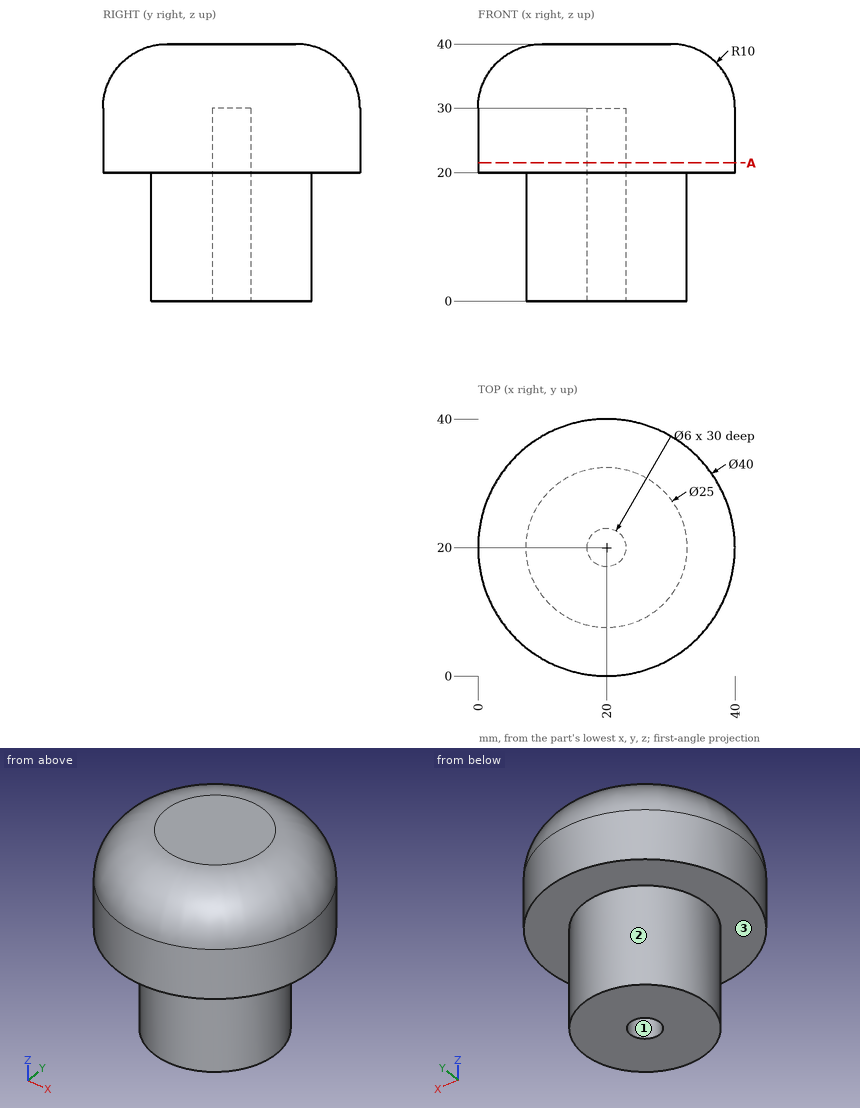
Answer from the drawing. Dimensions are ordinates in mm from the lowest x, y and z of the part. Give positions to 0.01 mm unless a question says otherwise; leave off trailing zeros. Order: outer loops, then holes, each group sorted by start corner. A loop starts at its lowest first (then second) coordinate and runs counter-clockwise, first axis right, second up. Notation, with made-up numbers: (80, 28.25) - (102, 28.25) arc R21 ccw to (102, 39.25) - close; hole circle Ø11 at (40.25, -38). An arc over 180 degrees is marked (long way). One line per item, written item: value. Start each with the question number.
1. For a pull along X with two mould halves and no side action, classify the marked faces 1, 2 and 3 as released by +X, released by -X, zero draft, split by the parting line, or undercut.
2. Consider line 1 (Y direction, x = 20, z = 18); line 2 (X direction, y = 17.5, z = 18.5); line 3 (X direction, y = 22, z = 28). Determine where each line is inside the solid, lowest interval first.
3. Each of these flat-tipped pins is pushed along its axis until it touches: pin 1 Ø1.5 at (y, z) = (17.5, 10.5) entering from -X; pin 2 Ø1 at (y, z) = (9.5, 32.5) entering from -X; pin 3 Ø2 at (x, z) = (26, 12) entering from +Y; pin 4 Ø20 at (x, y) = (18.5, 12.5) entering from -Z. Where does it stop, or does it pass through?
4. Section A-A, the plane z = 21.5 is taken. Write down the section's boundary in (x, y).
Filled sheet:
1. face 1: undercut
1. face 2: split by the parting line
1. face 3: zero draft
2. line 1: 7.5 to 17, 23 to 32.5
2. line 2: 7.75 to 18.34, 21.66 to 32.25
2. line 3: 0.1 to 17.76, 22.24 to 39.9
3. pin 1: x = 7.62
3. pin 2: x = 3.01
3. pin 3: y = 31.46
3. pin 4: z = 0
4. outline: circle Ø40 at (20, 20); hole circle Ø6 at (20, 20)
